Could you check a few things on this model? Use its own coordinates, in mm. A direction names the side the tool comes from. Coordinates: 2 decimals unless noted, no trailing zeros. Loops run counter-clockwise (first coordinate to the right, second up) from the corner with the lowest first, then second, coordinate; pieces in that order, holes last. Notation, with made-up numbers: (86, -18.75) -> (126, -18.75) arc R28 ccw to (126, 11.25) -> close; hole circle Ø8 at (-1.75, 34.5). An arc over 180 degrees is marked (long way). One line per question, with ' | ' between items.
Autodesk Inventor part; units mm, degrees
ref_plane "YZ Plane" through (0, 0, 0) normal (1, 0, 0) x (0, 1, 0)
ref_plane "XZ Plane" through (0, 0, 0) normal (0, 1, 0) x (-1, 0, 0)
ref_plane "XY Plane" through (0, 0, 0) normal (0, 0, 1) x (1, 0, 0)
sketch "Sketch1" plane through (0, 0, 0) normal (0, 0, 1) x (1, 0, 0)
  line L0 (-26.5191, 402.9946) -> (-1.1191, 402.9946)
  line L1 (-1.1191, 402.9946) -> (-1.1191, 352.1946)
  line L2 (-1.1191, 352.1946) -> (-26.5191, 352.1946)
  line L3 (-26.5191, 352.1946) -> (-26.5191, 402.9946)
  line L4 (-23.3441, 399.8196) -> (-4.2941, 399.8196)
  line L5 (-4.2941, 399.8196) -> (-4.2941, 355.3696)
  line L6 (-4.2941, 355.3696) -> (-23.3441, 355.3696)
  line L7 (-23.3441, 355.3696) -> (-23.3441, 399.8196)
  point P0 (0, 0)
  dimension "d0" = 50.8
  dimension "d1" = 25.4
  dimension "d2" = 3.175
extrude "Extrusion1" add sketch "Sketch1" along normal blind 546.1
sketch "Sketch2" plane through (0, 0, 0) normal (0, 0, -1) x (-1, 0, 0)
  circle A0 centre (13.8191, 377.5946) radius 12.7
  line L0 (23.3441, 399.8196) -> (23.3441, 355.3696)
  line L1 (23.3441, 355.3696) -> (4.2941, 355.3696)
  point P0 (0, 0)
  point P1 (23.3441, 377.5946)
  point P2 (13.8191, 355.3696)
  dimension "d6" = 25.4
extrude "Extrusion2" add sketch "Sketch2" along normal blind 25.4 and the other way blind 603.25
sketch "Sketch4" plane through (-26.5191, 352.1946, 0) normal (-1, 0, 0) x (0, 0, 1)
  circle A0 centre (60.325, 25.4) radius 7.9375
  line L0 (0, 25.4) -> (0, 50.8)
  circle A1 centre (485.775, 25.4) radius 7.9375
  line L1 (546.1, 0) -> (546.1, 25.4)
  line L2 (0, 25.4) -> (0, 0)
  point P0 (0, -352.1946)
  point P1 (273.05, 25.4)
  dimension "d17" = 15.875
  dimension "d19" = 15.875
  dimension "d23" = 546.1
  dimension "d24" = 273.05
  dimension "d26" = 212.725
  dimension "d27" = 425.45
extrude "Extrusion4" cut sketch "Sketch4" against normal through all
equation "\"d19\" = d17"
properties part number "Intake 3 Cross Bar"
Q1. We'd pull the mould along X, two halves only. Please class faces 5 (the face through (-23.344, 393, 269)), 6 (the face through (-14, 378, -25.4)), 7 (the face through (-1.119, 378, 269)): released by +X, released by -X, zero draft, split by the parting line, or undercut.
Values follow:
face 5: undercut | face 6: zero draft | face 7: released by +X
Q2. For faces 1 (the face through (-14, 399.82, 269)), 2 (the face through (-15, 355, 0)), 3 (the face through (-15, 355, 546.1)), 4 (the face through (-14, 378, 603.25)), which set-ups out of +Z, -Z, +X, -X, +Y, -Y let a thin tool reach every point of the face, with its end or its side?
Values follow:
face 1: +Z, -Z | face 2: -Z, -Y | face 3: +Z, -Y | face 4: +Z, +X, -X, +Y, -Y
Q3. Imagine slicing it at B-B on z = 136. Write out the boundary of the cut face in (x, y), plus the area to 3 significant figures.
Values follow:
outline: (-26.52, 352.19) -> (-1.12, 352.19) -> (-1.12, 402.99) -> (-26.52, 402.99) -> close; hole (-23.34, 355.37) -> (-4.29, 355.37) -> (-4.29, 369.19) arc R12.7 cw to (-23.34, 369.19) -> close; hole (-23.34, 385.99) arc R12.7 cw to (-4.29, 385.99) -> (-4.29, 399.82) -> (-23.34, 399.82) -> close | area: 877 mm2
Q4. Please list where these lines run through material, in increasing order: L1, parallel to Y at x = -23.25, z = 143.5; L2, parallel to Z at x = -22.5, y = 377.5; L3, parallel to X at y = 363, z = 468.5. Write a range as [from, to].
Values follow:
L1: y = [352.19, 355.37], [369.09, 386.1], [399.82, 402.99] | L2: z = [-25.4, 52.39], [68.26, 477.84], [493.71, 603.25] | L3: x = [-26.52, -23.34], [-4.29, -1.12]
Q5. Imagine slicing it at A-A on x = -11.75. Give the number of separate pieces and of enclosed holes in the cut face, plus the area to 3 significant figures.
Values follow:
separate pieces: 3 | enclosed holes: 2 | area: 18,800 mm2
